Model file for the job. Use its own axes, mm. Face numbers are marked on the shaded views. Coordinates: 2 decimals unless noted, no trailing zeros. Order: outer loops, then holes, each group sorted by start corner. A loop starts at its lowest first (then second) coordinate and runs counter-clockwise, first axis right, second up. Notation, with made-up numbers: (44.25, -35) -> (77.25, -35) arc R15 ccw to (77.25, -7) -> close; hole circle Ø2 at (46, 85.5). An arc over 180 degrees is marked (long way). Return JSON: item names as keys, results as strings. Group by question number.
1) Probe line 1 (Z direction, x = -15.5, y = 4.5); line 2 (Z direction, x = 16.25, y = 2); line 3 (X direction, y = 0, z = 29.5). List the from-to ranges inside material, lowest first.
2) Cut at C-C (x = -16.25). Write the cut outline in (y, z).
3) Pull direction X, two halves, no side cores. Call the marked faces 1 and 2: +X half, -X half, draft (parallel to the pull), parting line (faces both ways), or undercut.
4) Flat gauge pins, fed straight in: pin 1 (4 mm diameter, centred on x = -16.25, z = 28.15, fed in from -Y); pin 2 (5 mm diameter, centred on x = 13, z = -23, fed in from +Y); pin 3 (1.5 mm diameter, centred on x = 25.5, y = 2, fed in from +Z). Where does each tip first touch, or does it go through?
5) Cut at A-A (z = 0). Write the cut outline in (x, y), and give its area (3 significant figures).
6) Cut at D-D (z = 21.5). Write the cut outline in (x, y), and give its area (3 significant figures).
7) Cut at B-B (x = 0). Write the cut outline in (y, z), and give its area (3 significant figures).
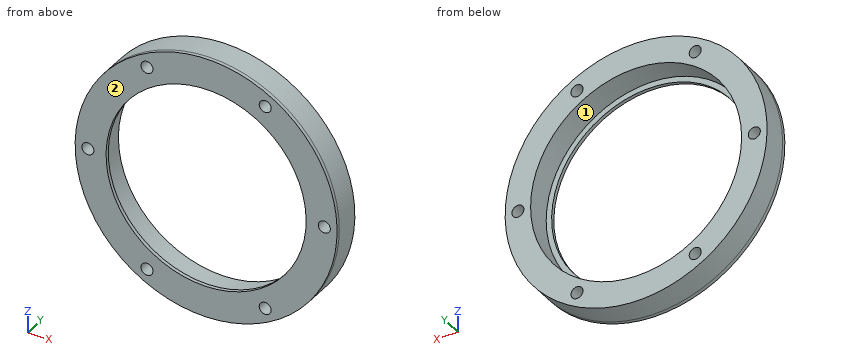
from build123d import *

# Parameters (mm, degrees)
SKETCH_2_R         = 36
SKETCH_2_R_2       = 29
EXTRUDE_1_DEPTH    = 7
EXTRUDE_START      = 1
SKETCH_3_R         = 36
SKETCH_3_R_2       = 27.5
EXTRUDE_2_DEPTH    = 1
HOLE_WIZARD_M4_1_D = 3.3


with BuildPart() as part:
    # 草图2 → 凸台-拉伸1 (new body)
    with BuildSketch(Plane(origin=(0, 0, 0), x_dir=(1, 0, 0), z_dir=(0, 1, 0))):
        with Locations(Location((0, 0, 0), (0, 0, 270))):
            Circle(SKETCH_2_R)
        with Locations(Location((0, 0, 0), (0, 0, 270))):
            Circle(SKETCH_2_R_2, mode=Mode.SUBTRACT)
    extrude(amount=EXTRUDE_1_DEPTH)

    # 草图3 → 凸台-拉伸2 (add)
    with BuildSketch(Plane.XZ.offset(EXTRUDE_START)):
        with Locations(Location((0, 0, 0), (0, 0, 270))):
            Circle(SKETCH_3_R)
        with Locations(Location((0, 0, 0), (0, 0, 270))):
            Circle(SKETCH_3_R_2, mode=Mode.SUBTRACT)
    extrude(amount=-EXTRUDE_2_DEPTH)

    # M4 螺纹孔1 (through all)
    with Locations(Plane(origin=(0, 7, 0), x_dir=(1, 0, 0), z_dir=(0, 1, 0))):
        with Locations((-16.25, 28.145825623), (16.25, 28.145825623), (32.5, 0), (16.25, -28.145825623), (-16.25, -28.145825623), (-32.5, 0)):
            Hole(HOLE_WIZARD_M4_1_D / 2)


solid = part.part
Answers below:
{
 "1": {"line 1": "z = -32.49 to -29.62, -26.68 to -24.51, 24.51 to 26.68, 29.62 to 32.49", "line 2": "z = -32.12 to -29.8, -26.5 to -24.02, 24.02 to 26.5, 29.8 to 32.12", "line 3": "x = -20.63 to -17.19, -15.31 to 15.31, 17.19 to 20.63"},
 "2": {"outline": "(-1, -32.12) -> (7, -32.12) -> (7, -29.8) -> (-1, -29.8) -> close; (-1, -26.5) -> (7, -26.5) -> (7, -24.02) -> (0, -24.02) -> (0, -22.19) -> (-1, -22.19) -> close; (-1, 22.19) -> (0, 22.19) -> (0, 24.02) -> (7, 24.02) -> (7, 26.5) -> (-1, 26.5) -> close; (-1, 29.8) -> (7, 29.8) -> (7, 32.12) -> (-1, 32.12) -> close"},
 "3": {"face 1": "undercut", "face 2": "draft"},
 "4": {"pin 1": "stops at y = -1", "pin 2": "stops at y = 0", "pin 3": "stops at z = 26.14"},
 "5": {"outline": "(-36, -1) -> (-34.15, -1) -> (-34.15, 7) -> (-36, 7) -> close; (-30.85, -1) -> (-27.5, -1) -> (-27.5, 0) -> (-29, 0) -> (-29, 7) -> (-30.85, 7) -> close; (27.5, -1) -> (30.85, -1) -> (30.85, 7) -> (29, 7) -> (29, 0) -> (27.5, 0) -> close; (34.15, -1) -> (36, -1) -> (36, 7) -> (34.15, 7) -> close", "area": "62.2 mm^2"},
 "6": {"outline": "(-28.87, -1) -> (-17.15, -1) -> (-17.15, 0) -> (-19.46, 0) -> (-19.46, 7) -> (-28.87, 7) -> close; (17.15, -1) -> (28.87, -1) -> (28.87, 7) -> (19.46, 7) -> (19.46, 0) -> (17.15, 0) -> close", "area": "155 mm^2"},
 "7": {"outline": "(-1, -36) -> (7, -36) -> (7, -29) -> (0, -29) -> (0, -27.5) -> (-1, -27.5) -> close; (-1, 27.5) -> (0, 27.5) -> (0, 29) -> (7, 29) -> (7, 36) -> (-1, 36) -> close", "area": "115 mm^2"}
}
